Drawing for the job (mm, zero at the part's lowest x, y, z). Give positions to 0.01 mm unless a question says otherwise; leave off trailing zeros. Order: outer loops, then holes, each group sorted by start corner. A loop starts at its lowest first (then second) coordinate and runs counter-clockwise, first axis right, second up. Notation, with made-up numbers: (78.5, -18.75) - (118.5, -18.75) arc R23 ccw to (118.5, 18.25) - close; hole circle Ø8 at (10.25, 29). An arc over 180 degrees is marked (long way). Write each question's results on one line, items separated by ' | '. Start each with the question number.
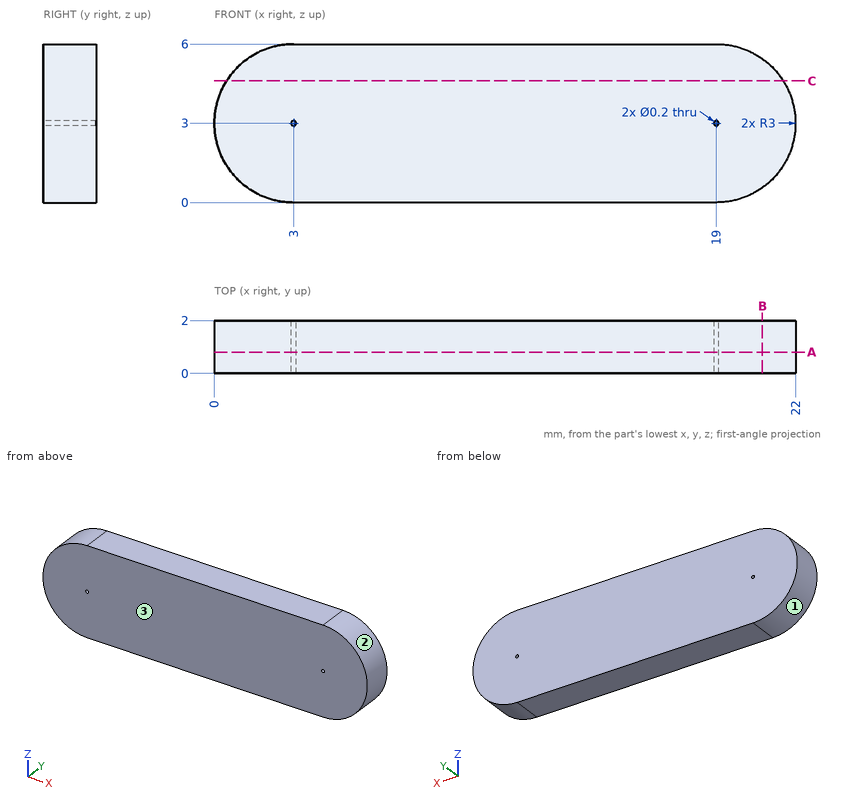
Item 1: Cut at B-B, the plane x = 20.75. List the corners of the cut face in (y, z), then the cut area to 3 significant figures.
Item 2: Two-plate mould, pull along X, no slides. Class the marked faces 1, 2 and 3: +X half, -X half, draft (parallel to the pull), parting line (faces both ways), or undercut.
Item 3: Cut at C-C, the plane z = 4.6. List the corners of the cut face in (x, y).
Item 4: Cut at A-A, the plane y = 0.8. List the corners of the cut face in (x, z).
Item 5: Probe line 1 along Z through (x, y) = (3, 1.5); line 2 along X through (y, z) = (0.1, 2.6); line 3 along X through (y, z) = (1.3, 3.7). List the from-to ranges inside material, lowest first. Write a range as from..to.
Values found:
1) outline: (0, 0.56) - (2, 0.56) - (2, 5.44) - (0, 5.44) - close | area: 9.75 mm2
2) face 1: -X half | face 2: +X half | face 3: draft
3) outline: (0.46, 0) - (21.54, 0) - (21.54, 2) - (0.46, 2) - close
4) outline: (3, 0) - (19, 0) arc R3 ccw to (19, 6) - (3, 6) arc R3 ccw to start; hole circle Ø0.2 at (3, 3); hole circle Ø0.2 at (19, 3)
5) line 1: z = 0..2.9, 3.1..6 | line 2: x = 0.03..21.97 | line 3: x = 0.08..21.92
